Geometry: final body of the model. Coordinates: model frame, mm. Face numbers are marked on the shaded views. A direction names the side the tool comes from. Give positions to 0.01 mm unless a question says otherwise; leave off trailing zeros. Order: outer loops, then holes, each group sorted by start corner. A loop starts at its lowest first (then second) coordinate and runs counter-clockwise, first axis right, second up. Notation, with made-up numbers: (75, 89) -> (116, 89) arc R11 ccw to (116, 103) -> close; hole circle Ø9 at (35, -38.75). An arc over 180 degrees is marked (long way). One line per question, with ' | ' between items.
from build123d import *

# Parameters (mm, degrees)
SKETCH1_W                     = 30.48
SKETCH1_H                     = 50.8
SKETCH1_R                     = 1.524
BOSS_EXTRUDE1_DEPTH           = 12.7
CUT_EXTRUDE1_DEPTH            = 55.536112806
SKETCH3_W                     = 13.253769435
SKETCH3_H                     = 10.922
CUT_EXTRUDE2_DEPTH            = 6.35
SKETCH4_W                     = 23.114
SKETCH4_H                     = 19.05
CUT_EXTRUDE3_DEPTH            = 3.175
CUT_EXTRUDE4_DEPTH            = 2.54
SKETCH7_W                     = 3.272
SKETCH7_H                     = 3.175
SKETCH7_W_2                   = 3.302
BOSS_EXTRUDE2_DEPTH           = 16.51
SKETCH8_W                     = 16.54
SKETCH8_H                     = 3.175
CUT_EXTRUDE5_DEPTH            = 38.438083551
CUT_EXTRUDE5_DEPTH_BACK       = 38.438083551
SKETCH9_W                     = 30.48
SKETCH9_H                     = 5.13
SKETCH9_R                     = 1.524
BOSS_EXTRUDE3_DEPTH           = 6.1
SKETCH10_W                    = 30.48
SKETCH10_H                    = 48.26
SKETCH10_R                    = 1.524
BOSS_EXTRUDE4_DEPTH           = 6.35
CUT_EXTRUDE7_DEPTH            = 53.178302004
CUT_EXTRUDE7_DEPTH_BACK       = 53.178302004
BOSS_EXTRUDE5_DEPTH           = 6.35
BOSS_EXTRUDE5_DRAFT           = 4
BOSS_EXTRUDE5_PROFILE_2_DEPTH = 6.35
BOSS_EXTRUDE5_PROFILE_2_DRAFT = 4
CUT_EXTRUDE8_DEPTH            = 42.448814217
SKETCH14_W                    = 6.35
SKETCH14_H                    = 31.75
SKETCH14_H_2                  = 37.338
BOSS_EXTRUDE6_DEPTH           = 5.08


with BuildPart() as part:
    # Sketch1 → Boss-Extrude1 (new body)
    with BuildSketch(Plane(origin=(0, 0, 0), x_dir=(1, 0, 0), z_dir=(0, 1, 0))):
        Rectangle(SKETCH1_W, SKETCH1_H)
        with Locations(Location((8.89, -22.86, 0), (0, 0, 270))):
            Circle(SKETCH1_R, mode=Mode.SUBTRACT)
        with Locations(Location((-8.89, -22.86, 0), (0, 0, 270))):
            Circle(SKETCH1_R, mode=Mode.SUBTRACT)
        with Locations((8.89, 22.86)):
            Circle(SKETCH1_R, mode=Mode.SUBTRACT)
        with Locations((-8.89, 22.86)):
            Circle(SKETCH1_R, mode=Mode.SUBTRACT)
        with Locations((8.89, 22.86)):
            Circle(SKETCH1_R)
        with Locations((-8.89, 22.86)):
            Circle(SKETCH1_R)
    extrude(amount=BOSS_EXTRUDE1_DEPTH)

    # Sketch2 → Cut-Extrude1 (cut, through all)
    with BuildSketch(Plane.XY.offset(25.4)):
        Polygon((8.89, 12.7), (-8.89, 12.7), (-8.89, 6.35), (-11.557, 6.35), (-11.557, 4.78), (11.557, 4.78), (11.557, 6.35), (8.89, 6.35), align=None)
    extrude(amount=-CUT_EXTRUDE1_DEPTH, mode=Mode.SUBTRACT)

    # Sketch3 → Cut-Extrude2 (cut)
    with BuildSketch(Plane(origin=(0, 12.7, 0), x_dir=(1, 0, 0), z_dir=(0, 1, 0))):
        Polygon((-15.24, -8.89), (-15.24, -25.4), (1.986230565, -25.4), (1.986230565, -14.478), (1.986230565, -8.89), align=None)
        with Locations((8.613115283, -19.939)):
            Rectangle(SKETCH3_W, SKETCH3_H)
    extrude(amount=-CUT_EXTRUDE2_DEPTH, mode=Mode.SUBTRACT)

    # Sketch4 → Cut-Extrude3 (cut)
    with BuildSketch(Plane(origin=(0, 4.78, 0), x_dir=(1, 0, 0), z_dir=(0, 1, 0))):
        with Locations((0, 15.875)):
            Rectangle(SKETCH4_W, SKETCH4_H)
    extrude(amount=-CUT_EXTRUDE3_DEPTH, mode=Mode.SUBTRACT)

    # Sketch6 → Cut-Extrude4 (cut)
    with BuildSketch(Plane(origin=(0, 0, -25.4), x_dir=(-1, 0, 0), z_dir=(0, 0, -1))):
        Polygon((11.557, 6.35), (11.557, 1.605), (-11.557, 1.605), (-11.557, 6.35), (-8.89, 6.35), (-8.89, 12.7), (-15.24, 12.7), (-15.24, 0), (15.24, 0), (15.24, 12.7), (8.89, 12.7), (8.89, 6.35), align=None)
    extrude(amount=-CUT_EXTRUDE4_DEPTH, mode=Mode.SUBTRACT)

    # Sketch7 → Boss-Extrude2 (add)
    with BuildSketch(Plane(origin=(0, 0, -6.35), x_dir=(-1, 0, 0), z_dir=(0, 0, -1))):
        with Locations((-9.921, 3.1925)):
            Rectangle(SKETCH7_W, SKETCH7_H)
        with Locations((9.906, 3.1925)):
            Rectangle(SKETCH7_W_2, SKETCH7_H)
    extrude(amount=BOSS_EXTRUDE2_DEPTH)

    # Sketch8 → Cut-Extrude5 (cut, two sides)
    with BuildSketch(Plane(origin=(0, 0, -6.35), x_dir=(-1, 0, 0), z_dir=(0, 0, -1))) as cut_extrude5_sk:
        with Locations((-0.015, 3.1925)):
            Rectangle(SKETCH8_W, SKETCH8_H)
    extrude(amount=CUT_EXTRUDE5_DEPTH, mode=Mode.SUBTRACT)
    extrude(cut_extrude5_sk.sketch, amount=-CUT_EXTRUDE5_DEPTH_BACK, mode=Mode.SUBTRACT)

    # Sketch9 → Boss-Extrude3 (add)
    with BuildSketch(Plane.XZ):
        with Locations((0, 22.835)):
            Rectangle(SKETCH9_W, SKETCH9_H)
        with Locations(Location((-8.89, 22.86, 0), (0, 0, 270))):
            Circle(SKETCH9_R, mode=Mode.SUBTRACT)
        with Locations(Location((8.89, 22.86, 0), (0, 0, 270))):
            Circle(SKETCH9_R, mode=Mode.SUBTRACT)
        with Locations((0, -20.295)):
            Rectangle(SKETCH9_W, SKETCH9_H)
    extrude(amount=BOSS_EXTRUDE3_DEPTH)

    # Sketch10 → Boss-Extrude4 (add)
    with BuildSketch(Plane.XZ.offset(6.1)):
        with Locations((0, 1.27)):
            Rectangle(SKETCH10_W, SKETCH10_H)
        with Locations(Location((8.89, 22.86, 0), (0, 0, 270))):
            Circle(SKETCH10_R, mode=Mode.SUBTRACT)
        with Locations(Location((-8.89, 22.86, 0), (0, 0, 270))):
            Circle(SKETCH10_R, mode=Mode.SUBTRACT)
    extrude(amount=BOSS_EXTRUDE4_DEPTH)

    # Sketch11 → Cut-Extrude7 (cut, two sides)
    with BuildSketch(Plane.XY.offset(25.4)) as cut_extrude7_sk:
        Polygon((-7.62, -12.45), (0, -12.45), (0, -7.7002), (-11.557, -7.7002), (-11.557, -9.275), (-7.62, -9.275), align=None)
        Polygon((0, -7.7002), (0, -12.45), (7.62, -12.45), (7.62, -9.275), (11.557, -9.275), (11.557, -7.7002), align=None)
    extrude(amount=CUT_EXTRUDE7_DEPTH, mode=Mode.SUBTRACT)
    extrude(cut_extrude7_sk.sketch, amount=-CUT_EXTRUDE7_DEPTH_BACK, mode=Mode.SUBTRACT)


with BuildPart() as boss_extrude5_tool:
    # Sketch12 → Boss-Extrude5 (with draft: the straight prism first)
    with BuildSketch(Plane(origin=(0, 0, -22.86), x_dir=(-1, 0, 0), z_dir=(0, 0, -1))):
        Polygon((-7.62, -12.45), (-7.62, -9.275), (-11.557, -9.275), (-15.24, -9.275), (-15.24, -12.45), align=None)
    extrude(amount=BOSS_EXTRUDE5_DEPTH)
    # Boss-Extrude5: the draft: its side faces are tilted about the plane it starts from
    boss_extrude5_sides = [boss_extrude5_tool.faces().sort_by_distance(p)[0] for p in [
        (7.62, -10.8625, -26.035),
        (15.24, -10.8625, -26.035),
        (11.43, -9.275, -26.035),
        (11.43, -12.45, -26.035),
    ]]
    draft(boss_extrude5_sides, Plane(origin=(0, 0, -22.86), x_dir=(-1, 0, 0), z_dir=(0, 0, -1)), BOSS_EXTRUDE5_DRAFT)


with BuildPart() as part_1:
    add(part.part)

    # Boss-Extrude5: add boss_extrude5_tool
    add(boss_extrude5_tool.part)


with BuildPart() as boss_extrude5_profile_2_tool:
    # Sketch12 → Boss-Extrude5 profile 2 (with draft: the straight prism first)
    with BuildSketch(Plane(origin=(0, 0, -22.86), x_dir=(-1, 0, 0), z_dir=(0, 0, -1))):
        Polygon((15.24, -12.45), (15.24, -9.275), (11.557, -9.275), (7.62, -9.275), (7.62, -12.45), align=None)
    extrude(amount=BOSS_EXTRUDE5_PROFILE_2_DEPTH)
    # Boss-Extrude5 profile 2: the draft: its side faces are tilted about the plane it starts from
    boss_extrude5_profile_2_sides = [boss_extrude5_profile_2_tool.faces().sort_by_distance(p)[0] for p in [
        (-11.43, -12.45, -26.035),
        (-11.43, -9.275, -26.035),
        (-15.24, -10.8625, -26.035),
        (-7.62, -10.8625, -26.035),
    ]]
    draft(boss_extrude5_profile_2_sides, Plane(origin=(0, 0, -22.86), x_dir=(-1, 0, 0), z_dir=(0, 0, -1)), BOSS_EXTRUDE5_PROFILE_2_DRAFT)


with BuildPart() as part_2:
    add(part_1.part)

    # Boss-Extrude5 profile 2: add boss_extrude5_profile_2_tool
    add(boss_extrude5_profile_2_tool.part)

    # Sketch13 → Cut-Extrude8 (cut, through all)
    with BuildSketch(Plane.XZ.offset(12.45)):
        Polygon((-22.129268927, 18.728628624), (-23.925320151, 20.524679849), (-15.843089642, 28.606910358), (-14.047038418, 26.810859133), (-11.837895412, 29.020002139), (-10.670462117, 27.852568843), (-23.170978637, 15.352052323), (-24.338411933, 16.519485619), align=None)
        Polygon((23.170978637, 15.352052323), (24.338411933, 16.519485619), (22.129268927, 18.728628624), (23.925320151, 20.524679849), (15.843089642, 28.606910358), (14.047038418, 26.810859133), (11.837895412, 29.020002139), (10.670462117, 27.852568843), (13.12303096, 25.4), (15.24, 25.4), (15.24, 23.28303096), align=None)
        Polygon((13.12303096, 25.4), (15.24, 23.28303096), (15.24, 25.4), align=None)
    extrude(amount=-CUT_EXTRUDE8_DEPTH, mode=Mode.SUBTRACT)

    # Sketch14 → Boss-Extrude6 (add)
    with BuildSketch(Plane(origin=(0, 12.7, 0), x_dir=(1, 0, 0), z_dir=(0, 1, 0))):
        with Locations((-12.065, 6.985)):
            Rectangle(SKETCH14_W, SKETCH14_H)
        with Locations((12.065, 4.191)):
            Rectangle(SKETCH14_W, SKETCH14_H_2)
    extrude(amount=BOSS_EXTRUDE6_DEPTH)


solid = part_2.part
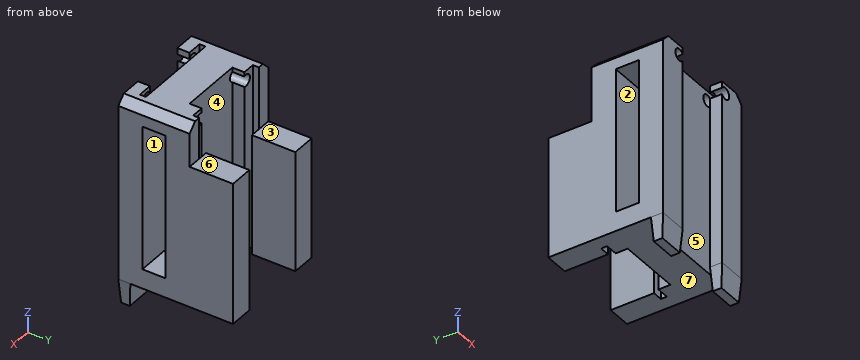
1) Set-up query: the marked faces 5, 6 and 7. Return all of +Z, -Z, +X, -X, +Y, -Y with unobstructed straight access to the full face (end or side cutting, diameter ignored); none if empty.
Check result:
face 5: +Z, -Z | face 6: +Z, +X, -X, +Y | face 7: -Z, +X, -X, +Y
2) Section A-A on y = -4.5. Return loops of the section in (x, z), plus the area to 3 significant figures.
Check result:
outline: (-15.24, -22.86) -> (15.24, -22.86) -> (15.24, -17.73) -> (-15.24, -17.73) -> close; (-15.24, 20.27) -> (15.24, 20.27) -> (15.24, 23.28) -> (13.12, 25.4) -> (-13.12, 25.4) -> (-15.24, 23.28) -> close; hole circle Ø3.05 at (-8.89, 22.86); hole circle Ø3.05 at (8.89, 22.86) | area: 294 mm^2
3) Pull-direction query (Z, two-part tool) for the marked faces 1, 2, 3 and 4; classes: +Z half, -Z half, draft (parallel to the pull), parting line (faces both ways), or undercut.
Check result:
face 1: undercut | face 2: undercut | face 3: +Z half | face 4: draft
4) Section C-C on x = -5.5. Return loops of the section in (y, z) (3 decimals).
Check result:
outline: (-7.7, -22.86) -> (1.605, -22.86) -> (1.605, 25.4) -> (-7.7, 25.4) -> close; hole (-6.1, -17.73) -> (0, -17.73) -> (0, 20.27) -> (-6.1, 20.27) -> close
5) Section D-D on z = -19.5. Return loops of the section in (x, y) (3 decimals).
Check result:
outline: (-15.24, -12.45) -> (-7.62, -12.45) -> (-7.62, -9.275) -> (-11.557, -9.275) -> (-11.557, -7.7) -> (11.557, -7.7) -> (11.557, -9.275) -> (7.62, -9.275) -> (7.62, -12.45) -> (15.24, -12.45) -> (15.24, 17.78) -> (8.89, 17.78) -> (8.89, 6.35) -> (11.557, 6.35) -> (11.557, 4.78) -> (8.285, 4.78) -> (8.285, 1.605) -> (-8.255, 1.605) -> (-8.255, 4.78) -> (-11.557, 4.78) -> (-11.557, 6.35) -> (-8.89, 6.35) -> (-8.89, 17.78) -> (-15.24, 17.78) -> close
6) Contact query for flat-ended pins moving along their axis: pin 1 Ø4 at (x, z) = (-14, 14) entering from +Y; pin 2 Ø7 at (x, y) = (13, 12) entering from +Z; pin 3 Ø5 at (x, z) = (8.89, 22.86) entering from +Y. Output: stop coordinate, or through.
Check result:
pin 1: stops at y = 6.35 | pin 2: stops at z = 14.48 | pin 3: stops at y = 4.78
7) Section B-B on z = 17. Return loops of the section in (x, y) (3 decimals).
Check result:
outline: (-15.24, -12.45) -> (-7.62, -12.45) -> (-7.62, -9.275) -> (-11.557, -9.275) -> (-11.557, -7.7) -> (11.557, -7.7) -> (11.557, -9.275) -> (7.62, -9.275) -> (7.62, -12.45) -> (15.24, -12.45) -> (15.24, -6.1) -> (-15.24, -6.1) -> close; (-15.24, 0) -> (15.24, 0) -> (15.24, 6.35) -> (11.557, 6.35) -> (11.557, 4.78) -> (8.285, 4.78) -> (8.285, 1.605) -> (-8.255, 1.605) -> (-8.255, 4.78) -> (-11.557, 4.78) -> (-11.557, 6.35) -> (-15.24, 6.35) -> close
8) Material intervals for probe 1 along X at (y, z) = (-4.75, 22.86); probe 2 along Z at (x, y) = (8.89, -10.45); probe 3 along Z at (x, y) = (8.89, 1.75), sorted ascending. Write a range as from..to.
Check result:
probe 1: x = -15.24..-10.41, -7.37..7.37, 10.41..15.24 | probe 2: z = -29.21..21.34, 24.38..25.4 | probe 3: z = -22.86..21.34, 24.38..25.4
